For this review, take the finished solid that the model builds, in its own axes (mm). A direction names the side the tool comes from. Round coordinates to 2 decimals unless told otherwise and drop trailing zeros. Loops run counter-clockwise (first coordinate to the right, second up) from the corner with the lowest first, then second, coordinate; pieces in that order, holes last.
1. Tool access review of faces 1 (the cylindrical face through (7.98, 8.26, 0.98)), 2 (the flat face through (5, 5, 0)), 3 (the flat face through (8, 23, 1.9)): name each direction out of +Z, -Z, +X, -X, +Y, -Y from which nothing blocks a thin tool from reaching the whole face with its end or side.
2. Consider section D-D on y = 2. State the section outline as (x, z) points.
3. Consider section A-A on x = 0. State the section outline as (y, z) points.
4. Consider section B-B on y = 14. State the section outline as (x, z) points, then the cut area to 3 significant figures.
5. Consider section C-C on z = 4.75. State the section outline as (x, y) points, then the cut area to 3 significant figures.
6. To check wall thickness, follow line 1 along Z through (x, y) = (5, 3.3); line 2 along Y through (x, z) = (7.5, -2); line 3 along Y through (x, z) = (9, 6). State the ranges of each line that lie inside material, in increasing order.
7. Clearance check with flat-ended pins moving along their axes: pin 1 Ø2 at (x, y) = (-8, 24) entering from +Z; pin 2 Ø2 at (x, y) = (7.5, 7.5) entering from +Z; pin 3 Ø1.5 at (y, z) = (23.5, 3) entering from +X; pin 4 Ø1.5 at (x, z) = (7.5, 5) entering from +Y. State where each tip first meets the part, or that it passes through.
8. Draft analysis for pull direction X (two halves, no side actions). For faces 4 (the flat face through (8, 21, 4)), 5 (the cylindrical face through (-7.62, 8.39, 0.98)), 6 (the flat face through (6, 24, 4)), 7 (the cylindrical face through (-6.285, 21.301, 4.365)), state which applies: released by +X, released by -X, zero draft, split by the parting line, or undercut.
Autodesk Inventor part; units mm, degrees
ref_plane "YZ Plane" through (0, 0, 0) normal (1, 0, 0) x (0, 1, 0)
ref_plane "XZ Plane" through (0, 0, 0) normal (0, 1, 0) x (-1, 0, 0)
ref_plane "XY Plane" through (0, 0, 0) normal (0, 0, 1) x (1, 0, 0)
sketch "Sketch1" plane through (0, 0, 0) normal (0, 1, 0) x (-1, 0, 0)
  line L0 (-10, -6.9) -> (10, -6.9)
  line L1 (10, -6.9) -> (10, 6.9)
  line L2 (10, 6.9) -> (-10, 6.9)
  line L3 (-10, 6.9) -> (-10, -6.9)
  line L4 (-10, -6.9) -> (10, 6.9) construction
  line L5 (10, -6.9) -> (-10, 6.9) construction
  point P0 (0, 0)
  dimension "d0" = 20
  dimension "d1" = 13.8
extrude "Extrusion1" add sketch "Sketch1" along normal blind 25
sketch "Sketch2" plane through (-10, 0, 6.9) normal (0, 0, 1) x (1, 0, 0)
  circle A0 centre (10, 14) radius 8.5
  circle A1 centre (2.5, 7.5) radius 0.9
  circle A2 centre (17.5, 7.5) radius 0.9
  point P0 (10, 0)
  dimension "d14" = 17
  dimension "d18" = 1.8
  dimension "d21" = 1.8
extrude "Extrusion2" cut sketch "Sketch2" against normal through all contours A0
sketch "Sketch3" plane through (-10, 0, 6.9) normal (0, 0, 1) x (1, 0, 0)
  circle A0 centre (10, 14) radius 8.5
  circle A1 centre (2.5, 7.5) radius 0.9
  circle A2 centre (17.5, 7.5) radius 0.9
  point P0 (10, 0)
  point P1 (10, 0)
  dimension "d24" = 17
  dimension "d25" = 1.8
  dimension "d26" = 1.8
extrude "Extrusion3" cut sketch "Sketch3" against normal blind 12 contours A1 | A2
sketch "Sketch5" plane through (-10, 0, 6.9) normal (0, 0, 1) x (1, 0, 0)
  circle A0 centre (2.5, 7.5) radius 0.9
  circle A1 centre (17.5, 7.5) radius 0.9
  circle A2 centre (10, 14) radius 8.5
  line L0 (0, 0) -> (20, 0)
  line L1 (20, 0) -> (20, 25)
  line L2 (0, 25) -> (20, 25)
  line L3 (0, 0) -> (0, 25)
  line L4 (10, 0) -> (10, 5)
  line L5 (0, 25) -> (4, 25)
  line L6 (4, 25) -> (4, 21)
  line L7 (4, 21) -> (0, 21)
  line L8 (20, 25) -> (16, 25)
  line L9 (0, 25) -> (20, 25)
  line L10 (16, 25) -> (16, 21)
  line L11 (16, 21) -> (20, 21)
  line L12 (20, 25) -> (20, 21)
  line L13 (20, 0) -> (20, 25)
  line L14 (0, 25) -> (4, 25)
  line L15 (4, 25) -> (4, 21)
  line L16 (4, 21) -> (0, 21)
  line L17 (0, 21) -> (0, 25)
  line L18 (16, 25) -> (20, 25)
  line L19 (20, 25) -> (20, 21)
  line L20 (20, 21) -> (16, 21)
  line L21 (16, 21) -> (16, 25)
  dimension "d33" = 5
  dimension "d38" = 4
  dimension "d39" = 4
  dimension "d40" = 4
extrude "Extrusion4" cut sketch "Sketch5" against normal blind 5 contours L3 L2 L6 L7 | L11 L10 L2 L1
fillet "Fillet1" radius 1 2 edges at (-6, 21, 4.4) (6, 21, 4.4)
sketch "Sketch6" plane through (0, 0, 0) normal (0, -1, 0) x (1, 0, 0)
  circle A0 centre (-5, 0) radius 1.4
  circle A1 centre (5, 0) radius 1.4
  point P0 (0, 0)
  dimension "d46" = 2.8
  dimension "d47" = 2.8
extrude "Extrusion5" cut sketch "Sketch6" against normal blind 5
properties part number "Sonar Mount" material "ABS Plastic"
Resolved:
1. face 1: +Z
1. face 2: -Y
1. face 3: +Z, +X, +Y
2. outline: (-10, -6.9) - (10, -6.9) - (10, 6.9) - (-10, 6.9) - close; hole circle Ø2.8 at (-5, 0); hole circle Ø2.8 at (5, 0)
3. outline: (0, -6.9) - (5.5, -6.9) - (5.5, 6.9) - (0, 6.9) - close; (22.5, -6.9) - (25, -6.9) - (25, 6.9) - (22.5, 6.9) - close
4. outline: (-10, -6.9) - (-8.5, -6.9) - (-8.5, 6.9) - (-10, 6.9) - close; (8.5, -6.9) - (10, -6.9) - (10, 6.9) - (8.5, 6.9) - close
4. area: 41.4 mm2
5. outline: (-10, 0) - (10, 0) - (10, 21) - (7, 21) arc R1 cw to (6, 22) - (6, 25) - (-6, 25) - (-6, 22) arc R1 cw to (-7, 21) - (-10, 21) - close; hole circle Ø17 at (0, 14); hole circle Ø1.8 at (-7.5, 7.5); hole circle Ø1.8 at (7.5, 7.5)
5. area: 236 mm2
6. line 1: z = -6.9 to -1.4, 1.4 to 6.9
6. line 2: y = 0 to 6.6, 8.4 to 10, 18 to 25
6. line 3: y = 0 to 21
7. pin 1: stops at z = 1.9
7. pin 2: stops at z = 6.9
7. pin 3: stops at x = 6
7. pin 4: stops at y = 21.03
8. face 4: zero draft
8. face 5: undercut
8. face 6: released by +X
8. face 7: released by -X
